Autodesk Inventor part; units mm, degrees
ref_plane "YZ Plane" through (0, 0, 0) normal (1, 0, 0) x (0, 1, 0)
ref_plane "XZ Plane" through (0, 0, 0) normal (0, 1, 0) x (-1, 0, 0)
ref_plane "XY Plane" through (0, 0, 0) normal (0, 0, 1) x (1, 0, 0)
sketch "Boceto1" plane through (0, 0, 0) normal (0, 1, 0) x (-1, 0, 0)
  circle A0 centre (0, 0) radius 80
  circle A1 centre (0, 0) radius 52.5
  dimension "d0" = 160
  dimension "d4" = 105
extrude "Extrusión1" add sketch "Boceto1" along normal blind 25 draft 50 contours A1
shell "Vaciado1" thickness 3 removed faces 1 at (12.2178, 25, 3.7687)
properties part number "Cuenco"
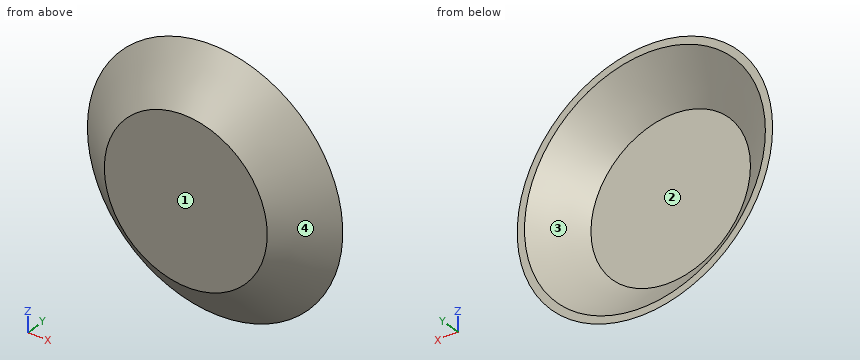
Work out the finished part from the listing and answer in its coordinate system (mm). Face numbers are marked on the shaded views. Round coordinates to 2 decimals unless told otherwise and drop trailing zeros. Write each loop counter-clockwise with the first axis right and the second up, starting at its lowest first coordinate (ties: lowest second). Pieces come first, ordered by that corner, then holes.
1) A cutting plane is placed at B-B on z = 0. Determine the outline of the cut face in (x, y), and give its area (3 significant figures).
2) Flat-ended cylindrical pins translate along their axes: P1, Ø8, axis at y = 22, z = 52.5, coming from the -X side; P2, Ø10, axis at x = -57.5, y = 21, coming from the +Z side; P3, Ø8, axis at y = 10, z = -49, coming from the -X side. Find the tip coordinate at first contact, or state that the pin passes through.
3) Determine the mould class of the marked faces 1, 2, 3 and 4 for opening direction Z: pulls with the +Z half, pulls with the -Z half, needs draft (parallel to the pull), parting line crosses it, or undercut.
4) A cutting plane is placed at A-A on x = 0. Determine the outline of the cut face in (y, z), and give its area (3 significant figures).
5) A cutting plane is placed at C-C on y = 19.5. Determine the outline of the cut face in (x, z).
6) Consider probe 1 along Z at (x, y) = (64, 23.25); probe 2 along Z at (x, y) = (40.5, 3.5); probe 3 along Y at (x, z) = (-37.5, -27). Determine where each line is inside the solid, lowest interval first.
Entries:
1. outline: (-82.29, 25) - (-52.5, 0) - (52.5, 0) - (82.29, 25) - (77.63, 25) - (51.41, 3) - (-51.41, 3) - (-77.63, 25) - close
1. area: 531 mm2
2. P1: stops at x = -65.47
2. P2: stops at z = 61.66
2. P3: stops at x = -49.9
3. face 1: needs draft
3. face 2: undercut
3. face 3: undercut
3. face 4: parting line crosses it
4. outline: (0, -52.5) - (25, -82.29) - (25, -77.63) - (3, -51.41) - (3, 51.41) - (25, 77.63) - (25, 82.29) - (0, 52.5) - close
4. area: 531 mm2
5. outline: circle Ø151.48 at (0, 0); hole circle Ø142.14 at (0, 0)
6. probe 1: z = -48.35 to -40.13, 40.13 to 48.35
6. probe 2: z = -39.64 to -32.62, 32.62 to 39.64
6. probe 3: y = 0 to 3
